Design review of the part built by this model. Coordinates are the model's own, in mm. Face numbers are marked on the shaded views. A direction names the side the tool comes from. Coordinates: 2 decimals unless noted, no trailing zeros. Loops run counter-clockwise (first coordinate to the right, second up) from the corner with the lowest first, then second, coordinate; pieces in that order, holes last.
Q1. Machinability: for the marked faces 5, 6 and 7, which of the approach directions +Z, -Z, +X, -X, +Y, -Y give a long, thin tool a straight path to every point of the face, cutting with its end or side? Answer none if there is none.
Q2. Add section C-C on z = 6.5. Give the boundary of the cut face in (x, y), and give its area (3 significant figures).
Q3. Add section A-A on x = -75. Give the boundary of the cut face in (y, z), and give its area (4 significant figures).
Q4. Add section D-D on x = -33. Give the boundary of the cut face in (y, z), and give its area (3 significant figures).
Q5. Add section B-B on y = -19. Give the boundary of the cut face in (x, z), and give its area (3 significant figures).
Q6. Wall thickness on probe 1 along Z at (x, y) = (75, -7.5); probe 2 along Z at (x, y) = (-55.5, -10); probe 3 along X at (y, z) = (-4.5, -3): over which ranges is each line inside the solid? List them lowest first.
Q7. For P1, Ø6, axis at x = -23, y = -43, coming from the +Z side; P2, Ø11.5, axis at x = -73.5, z = 8, coming from the -Y side; P3, Ø5, axis at y = -45.5, z = 7.5, coming from the -X side; P4, Ø4, axis at x = 67, z = -2.5, coming from the +Y side, all flat-tipped, find the tip position at first contact; note any pin that passes through.
Q8. Draft analysis for pull direction Z (two halves, no side actions). For the marked faces 1, 2, 3 and 4, state which applies: released by +Z, released by -Z, zero draft, split by the parting line, or undercut.
```python
from build123d import *

# Parameters (mm, degrees)
DODANIE_WYCI_GNI_CIE1_DEPTH = 14.5
DODANIE_WYCI_GNI_CIE2_START = 3
DODANIE_WYCI_GNI_CIE2_DEPTH = 3
DODANIE_WYCI_GNI_CIE3_DEPTH = 3
OTW_R_10_0_10_1_D           = 10
WYTNIJ_WYCI_GNI_CIE1_START  = -0.5
SZKIC7_W                    = 25
SZKIC7_H                    = 29
SZKIC7_R                    = 5
WYTNIJ_WYCI_GNI_CIE1_DEPTH  = 0.5


with BuildPart() as part:
    # Szkic1 → Dodanie-wyciągnięcie1 (new, symmetric)
    with BuildSketch(Plane.XY):
        with BuildLine():
            Line((-83, -10), (-68.373971656, -10))
            ThreePointArc((-68.373971656, -10), (-65.240055803, -11.104031388), (-63.490116538, -13.928571429))
            ThreePointArc((-63.490116538, -13.928571429), (0, -65), (63.490116538, -13.928571429))
            ThreePointArc((63.490116538, -13.928571429), (65.240055803, -11.104031388), (68.373971656, -10))
            Line((68.373971656, -10), (83, -10))
            Line((83, -10), (85, -8))
            Line((85, -8), (85, 0))
            Line((85, 0), (65, 0))
            Line((65, 0), (60, 0))
            ThreePointArc((60, 0), (0, -60), (-60, 0))
            Line((-60, 0), (-65, 0))
            Line((-65, 0), (-85, 0))
            Line((-85, 0), (-85, -8))
            Line((-85, -8), (-83, -10))
        make_face()
    extrude(amount=DODANIE_WYCI_GNI_CIE1_DEPTH, both=True)

    # Szkic2 → Dodanie-wyciągnięcie2 (add)
    with BuildSketch(Plane.XY.offset(14.5).offset(DODANIE_WYCI_GNI_CIE2_START)):
        with BuildLine():
            Line((-65, 0), (-60, 0))
            Line((-60, 0), (-53, 0))
            ThreePointArc((-53, 0), (0, -53), (53, 0))
            Line((53, 0), (60, 0))
            Line((60, 0), (65, 0))
            Line((65, 0), (85, 0))
            Line((85, 0), (85, -8))
            Line((85, -8), (83, -10))
            Line((83, -10), (68.373971656, -10))
            ThreePointArc((68.373971656, -10), (65.240055803, -11.104031388), (63.490116538, -13.928571429))
            ThreePointArc((63.490116538, -13.928571429), (0, -65), (-63.490116538, -13.928571429))
            ThreePointArc((-63.490116538, -13.928571429), (-65.240055803, -11.104031388), (-68.373971656, -10))
            Line((-68.373971656, -10), (-83, -10))
            Line((-83, -10), (-85, -8))
            Line((-85, -8), (-85, 0))
            Line((-85, 0), (-65, 0))
        make_face()
    extrude(amount=-DODANIE_WYCI_GNI_CIE2_DEPTH)

    # Szkic3 → Dodanie-wyciągnięcie3 (add)
    with BuildSketch(Plane(origin=(0, 0, -14.5), x_dir=(-1, 0, 0), z_dir=(0, 0, -1))):
        with BuildLine():
            Line((-65, 0), (-60, 0))
            Line((-60, 0), (-53, 0))
            ThreePointArc((-53, 0), (0, -53), (53, 0))
            Line((53, 0), (60, 0))
            Line((60, 0), (65, 0))
            Line((65, 0), (85, 0))
            Line((85, 0), (85, -8))
            Line((85, -8), (83, -10))
            Line((83, -10), (68.373971656, -10))
            ThreePointArc((68.373971656, -10), (65.240055803, -11.104031388), (63.490116538, -13.928571429))
            ThreePointArc((63.490116538, -13.928571429), (0, -65), (-63.490116538, -13.928571429))
            ThreePointArc((-63.490116538, -13.928571429), (-65.240055803, -11.104031388), (-68.373971656, -10))
            Line((-68.373971656, -10), (-83, -10))
            Line((-83, -10), (-85, -8))
            Line((-85, -8), (-85, 0))
            Line((-85, 0), (-65, 0))
        make_face()
    extrude(amount=DODANIE_WYCI_GNI_CIE3_DEPTH)

    # Otwór Ø10.0 (10)1 (through all)
    with Locations(Plane(origin=(0, 0, 0), x_dir=(1, 0, 0), z_dir=(0, 1, 0))):
        with Locations((75, 0), (-75, 0)):
            Hole(OTW_R_10_0_10_1_D / 2)

    # Szkic7 → Wytnij-wyciągnięcie1 (cut)
    # profile 1 of 2: a face of its own
    with BuildSketch(Plane(origin=(0, 0, 0), x_dir=(1, 0, 0), z_dir=(0, 1, 0)).offset(WYTNIJ_WYCI_GNI_CIE1_START)):
        with Locations((-72.5, 0)):
            Rectangle(SZKIC7_W, SZKIC7_H)
        with Locations(Location((-75, 0, 0), (0, 0, 270))):
            Circle(SZKIC7_R, mode=Mode.SUBTRACT)
    # profile 2 of 2: a face of its own
    with BuildSketch(Plane(origin=(0, 0, 0), x_dir=(1, 0, 0), z_dir=(0, 1, 0)).offset(WYTNIJ_WYCI_GNI_CIE1_START)):
        with Locations((72.5, 0)):
            Rectangle(SZKIC7_W, SZKIC7_H)
    extrude(amount=WYTNIJ_WYCI_GNI_CIE1_DEPTH, mode=Mode.SUBTRACT)


solid = part.part
```
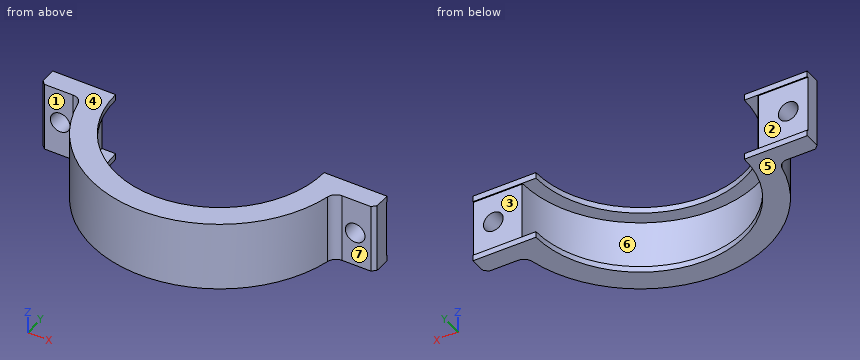
Entries:
1. face 5: -Z, +X, -X, +Y, -Y
1. face 6: +Y
1. face 7: +Z, -Z, +X, -Y
2. outline: (-85, -8) - (-83, -10) - (-68.37, -10) arc R5 cw to (-63.49, -13.93) arc R65 ccw to (63.49, -13.93) arc R5 cw to (68.37, -10) - (83, -10) - (85, -8) - (85, -0.5) - (60, -0.5) - (60, 0) arc R60 cw to (-60, 0) - (-60, -0.5) - (-85, -0.5) - close
2. area: 1,360 mm2
3. outline: (-10, -17.5) - (0, -17.5) - (0, -14.5) - (-0.5, -14.5) - (-0.5, -5) - (-10, -5) - close; (-10, 5) - (-0.5, 5) - (-0.5, 14.5) - (0, 14.5) - (0, 17.5) - (-10, 17.5) - close
3. area: 240.5 mm2
4. outline: (-56, -17.5) - (-41.47, -17.5) - (-41.47, -14.5) - (-50.11, -14.5) - (-50.11, 14.5) - (-41.47, 14.5) - (-41.47, 17.5) - (-56, 17.5) - close
4. area: 258 mm2
5. outline: (-62.16, -17.5) - (-49.48, -17.5) - (-49.48, -14.5) - (-56.91, -14.5) - (-56.91, 14.5) - (-49.48, 14.5) - (-49.48, 17.5) - (-62.16, 17.5) - close; (49.48, -17.5) - (62.16, -17.5) - (62.16, 17.5) - (49.48, 17.5) - (49.48, 14.5) - (56.91, 14.5) - (56.91, -14.5) - (49.48, -14.5) - close
5. area: 457 mm2
6. probe 1: z = -17.5 to -5, 5 to 17.5
6. probe 2: z = -17.5 to -14.5, 14.5 to 17.5
6. probe 3: x = -85 to -79, -71 to -59.83, 59.83 to 71, 79 to 85
7. P1: passes through
7. P2: stops at y = -10.04
7. P3: stops at x = -48.74
7. P4: stops at y = -0.5
8. face 1: zero draft
8. face 2: undercut
8. face 3: undercut
8. face 4: released by +Z
